Part model, mm, in its own coordinate system. A direction names the side the tool comes from. Give positions to 0.01 mm unless a question says otherwise; leave off trailing zeros. Order: outer loops, then holes, each group sorted by start corner. A loop starts at its lowest first (then second) coordinate and runs counter-clockwise, first axis right, second up. Notation, with made-up numbers: M 36,86 L 48,86 A23 cw 48,95 Z; hole C 10,-1 d5. An arc over 180 degrees is marked long. Return JSON: item names as keys, results as strings.
from build123d import *

# Parameters (mm, degrees)
SKETCH3_R           = 7.5
BOSS_EXTRUDE1_DEPTH = 8
BOSS_EXTRUDE2_DEPTH = 5
SKETCH5_W           = 56
SKETCH5_H           = 80
BOSS_EXTRUDE3_DEPTH = 5
SCALE1_SCALE        = 0.5


with BuildPart() as part:
    # Sketch1 → Revolve1 (revolve)
    with BuildSketch(Plane.XY):
        Polygon((-40, 60), (0, 60), (0, 50.773502692), (-10, 40.773502692), (-10, 15.773502692), (0, 10), (0, 0), (-40, 0), (-40, 10), (-30, 15.773502692), (-30, 40.773502692), (-40, 50.773502692), align=None)
    revolve(axis=Axis((0, 0, 0), (-1, 0, 0)))

    # Sketch3 → Boss-Extrude1 (add)
    with BuildSketch(Plane(origin=(0, 0, 0), x_dir=(0, 0, -1), z_dir=(1, 0, 0))):
        Circle(SKETCH3_R)
    boss_extrude1 = extrude(amount=BOSS_EXTRUDE1_DEPTH)

    # Sketch4 → Boss-Extrude2 (add)
    with BuildSketch(Plane(origin=(8, 0, 0), x_dir=(0, 0, -1), z_dir=(1, 0, 0))):
        with BuildLine():
            Line((8.84577787, 66.773419664), (88.84577787, 66.773419664))
            Line((88.84577787, 66.773419664), (23.828381591, -18.226580336))
            ThreePointArc((23.828381591, -18.226580336), (-17.50778863, -24.361390299), (-24.872723871, 16.773419664))
            Line((-24.872723871, 16.773419664), (8.84577787, 66.773419664))
        make_face()
    boss_extrude2 = extrude(amount=-BOSS_EXTRUDE2_DEPTH)

    # Mirror1: Boss-Extrude1, Boss-Extrude2 across plane
    add(boss_extrude1.mirror(Plane(origin=(-20, 0, 0), x_dir=(0, 0, 1), z_dir=(1, 0, 0))))
    add(boss_extrude2.mirror(Plane(origin=(-20, 0, 0), x_dir=(0, 0, 1), z_dir=(1, 0, 0))))

    # Sketch5 → Boss-Extrude3 (add)
    with BuildSketch(Plane(origin=(0, 66.773419664, 0), x_dir=(1, 0, 0), z_dir=(0, 1, 0))):
        with Locations((-20, 48.84577787)):
            Rectangle(SKETCH5_W, SKETCH5_H)
    extrude(amount=-BOSS_EXTRUDE3_DEPTH)


with BuildPart() as part_1:
    # Scale1: scaled about (-20, 6.593417993, -5.351287219)
    add(part.part.scale(SCALE1_SCALE).moved(Location((-10, 3.296708997, -2.675643609))))


solid = part_1.part
Q1. Band-saw the part on D-D (y = 24.5). Give the number of separate pieces and of enclosed holes in the cut face, then the cut area to 3 significant figures.
Established:
{"separate pieces": "3", "enclosed holes": "0", "area": "890 mm²"}
Q2. Band-saw the part on B-B (z = -34.5). Give the cut face in (x, y).
Established:
{"outline": "M -34,20.21 L -31.5,20.21 L -31.5,34.18 L -8.5,34.18 L -8.5,20.21 L -6,20.21 L -6,36.68 L -34,36.68 Z"}
Q3. Band-saw the part on A-A (x = -28.25). Give the cut face in (y, z), then the cut area to 3 significant figures.
Established:
{"outline": "C 3.3,-2.68 d60; C 3.3,-2.68 d12.02; M 34.18,-47.1 L 36.68,-47.1 L 36.68,-7.1 L 34.18,-7.1 Z; hole C 3.3,-2.68 d47.27", "area": "1,290 mm²"}
Q4. Band-saw the part on C-C (x = -19.75). Give the cut face in (y, z), then the cut area to 3 significant figures.
Established:
{"outline": "C 3.3,-2.68 d60; M 34.18,-47.1 L 36.68,-47.1 L 36.68,-7.1 L 34.18,-7.1 Z", "area": "2,930 mm²"}
Q5. Two-plate mould, pull along X, no slides. Class faces 5 (the flat face through (-6, 13, -10)), 6 (the flat face through (-20, 35, -47.099)), 7 (the flat face through (-30, 26, -16)): +X half, -X half, draft (parallel to the pull), parting line (faces both ways), or undercut.
Established:
{"face 5": "+X half", "face 6": "draft", "face 7": "undercut"}
Q6. Pin check, flat tips, straight feed: pin 1 (6 mm diameter, centred on y = -12, z = 15.5, fed in from -X); pin 2 (24 mm diameter, centred on y = 7, z = -27, fed in from +X); pin 3 (3 mm diameter, centred on x = -20.5, y = -2.5, fed in from -Z); pin 4 (2 mm diameter, centred on y = -11, z = -20.5, fed in from +X). Stop position of each tip, or through.
Established:
{"pin 1": "stops at x = -30", "pin 2": "stops at x = -6", "pin 3": "stops at z = -32.37", "pin 4": "stops at x = -11.54"}
Q7. Probe line 1 along X through (y, z) = (-5, -12.5); line 2 along X through (y, z) = (29, -22.5); line 3 along X through (y, z) = (31, -9.5). List the from-to ranges inside material, lowest first.
Established:
{"line 1": "x = -34 to -31.5, -25 to -15, -8.5 to -6", "line 2": "x = -34 to -31.5, -8.5 to -6", "line 3": "x = -34 to -31.5, -30 to -10, -8.5 to -6"}
Q8. 3-axis set-ups, long thin cutter, end or side, ignore diameter. For faces 1 (the conical face through (-10.24, 8.2, -4.22)), 2 (the flat face through (-7.23, 24.01, 1.45)), 3 (the flat face through (-32.77, 24.01, 1.45)), 4 (the flat face through (-32.77, 14.46, -30.1)): which of +Z, -Z, +X, -X, +Y, -Y reach the whole face in a straight line?
Established:
{"face 1": "none", "face 2": "+Z, +X, +Y", "face 3": "+Z, -X, +Y", "face 4": "-Z, -X, -Y"}
